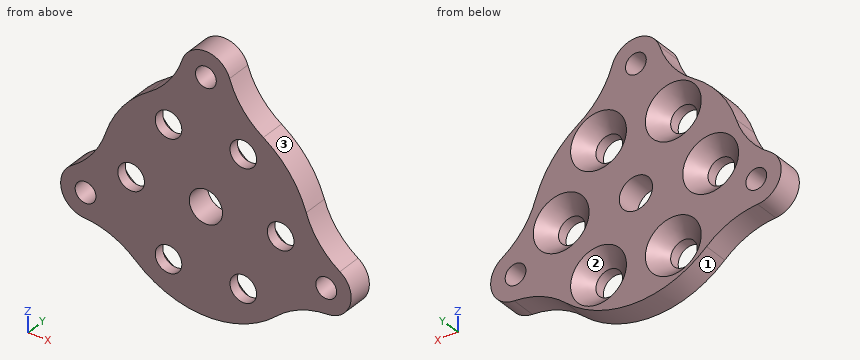
```python
from build123d import *

# Parameters (mm, degrees)
SKETCH1_R                    = 12.7
SKETCH1_R_2                  = 2
BOSS_EXTRUDE1_DEPTH          = 3
CSK_FOR_M3_SFHCS1_AT_2_COUNT = 2
CSK_FOR_M3_SFHCS1_AT_2_PITCH = 9
CSK_FOR_M3_SFHCS1_AT_3_COUNT = 2
CSK_FOR_M3_SFHCS1_AT_3_PITCH = 15.588457268
CSK_FOR_M3_SFHCS1_AT_4_COUNT = 2
CSK_FOR_M3_SFHCS1_AT_4_PITCH = 18
CSK_FOR_M3_SFHCS1_AT_5_COUNT = 2
CSK_FOR_M3_SFHCS1_AT_5_PITCH = 15.588457268
CSK_FOR_M3_SFHCS1_AT_6_COUNT = 2
CSK_FOR_M3_SFHCS1_AT_6_PITCH = 9
SKETCH6_R                    = 3
BOSS_EXTRUDE2_DEPTH          = 3
FILLET1_R                    = 10
TAP_DRILL_FOR_M3X0_5_TAP1_D  = 2.5


with BuildPart() as part:
    # Sketch1 → Boss-Extrude1 (new body)
    with BuildSketch(Plane(origin=(0, 0, 0), x_dir=(1, 0, 0), z_dir=(0, 1, 0))):
        with Locations(Location((0, 0, 0), (0, 0, 270))):
            Circle(SKETCH1_R)
        with Locations(Location((0, 0, 0), (0, 0, 270))):
            Circle(SKETCH1_R_2, mode=Mode.SUBTRACT)
    extrude(amount=BOSS_EXTRUDE1_DEPTH)

    # Sketch3 → CSK for M3 SFHCS1 (revolve, cut)
    with BuildSketch(Plane(origin=(-9, 3, 0), x_dir=(0, 0, 1), z_dir=(1, 0, 0))):
        Polygon((0, 0), (0, 3), (1.6, 3), (1.6, 1.76), (3.36, 0), align=None)
    csk_for_m3_sfhcs1 = revolve(axis=Axis((-9, 9.35, 0), (0, -1, 0)), mode=Mode.SUBTRACT)

    # CSK for M3 SFHCS1 at 2: CSK for M3 SFHCS1 ×2
    with Locations(*[Vector(0.5000000000000003, 0, -0.8660254037844386) * (i * CSK_FOR_M3_SFHCS1_AT_2_PITCH) for i in range(1, CSK_FOR_M3_SFHCS1_AT_2_COUNT)]):
        add(csk_for_m3_sfhcs1, mode=Mode.SUBTRACT)

    # CSK for M3 SFHCS1 at 3: CSK for M3 SFHCS1 ×2
    with Locations(*[Vector(0.8660254037844387, 0, -0.4999999999999999) * (i * CSK_FOR_M3_SFHCS1_AT_3_PITCH) for i in range(1, CSK_FOR_M3_SFHCS1_AT_3_COUNT)]):
        add(csk_for_m3_sfhcs1, mode=Mode.SUBTRACT)

    # CSK for M3 SFHCS1 at 4: CSK for M3 SFHCS1 ×2
    with Locations(*[(i * CSK_FOR_M3_SFHCS1_AT_4_PITCH, 0, 0) for i in range(1, CSK_FOR_M3_SFHCS1_AT_4_COUNT)]):
        add(csk_for_m3_sfhcs1, mode=Mode.SUBTRACT)

    # CSK for M3 SFHCS1 at 5: CSK for M3 SFHCS1 ×2
    with Locations(*[Vector(0.8660254037844387, 0, 0.49999999999999994) * (i * CSK_FOR_M3_SFHCS1_AT_5_PITCH) for i in range(1, CSK_FOR_M3_SFHCS1_AT_5_COUNT)]):
        add(csk_for_m3_sfhcs1, mode=Mode.SUBTRACT)

    # CSK for M3 SFHCS1 at 6: CSK for M3 SFHCS1 ×2
    with Locations(*[Vector(0.5000000000000002, 0, 0.8660254037844386) * (i * CSK_FOR_M3_SFHCS1_AT_6_PITCH) for i in range(1, CSK_FOR_M3_SFHCS1_AT_6_COUNT)]):
        add(csk_for_m3_sfhcs1, mode=Mode.SUBTRACT)

    # Sketch6 → Boss-Extrude2 (add)
    with BuildSketch(Plane(origin=(0, 3, 0), x_dir=(1, 0, 0), z_dir=(0, 1, 0))):
        with Locations((14.488887394, 3.882285677)):
            Circle(SKETCH6_R)
        with Locations((0, -15)):
            Circle(SKETCH6_R)
        with Locations((-14.488887394, 3.882285677)):
            Circle(SKETCH6_R)
    extrude(amount=-BOSS_EXTRUDE2_DEPTH)

    # Fillet1
    fillet1_edges = [part.edges().sort_by_distance(p)[0] for p in [
        (11.690211932, 1.5, -4.962755785),
        (12.605398401, 1.5, -1.547233383),
        (1.768004493, 1.5, 12.576333333),
        (-1.768004493, 1.5, 12.576333333),
        (-11.690211932, 1.5, -4.962755785),
        (-12.605398401, 1.5, -1.547233383),
    ]]
    fillet(fillet1_edges, radius=FILLET1_R)

    # Tap Drill for M3x0.5 Tap1 (through all)
    with Locations(Plane(origin=(0, 3, 0), x_dir=(1, 0, 0), z_dir=(0, 1, 0))):
        with Locations((-14.488887394, 3.882285677), (14.488887394, 3.882285677), (0, -15)):
            Hole(TAP_DRILL_FOR_M3X0_5_TAP1_D / 2)


solid = part.part
```
Design review of the part built by this model. Coordinates are the model's own, in mm. Face numbers are marked on the shaded views. Coordinates: 2 decimals unless noted, no trailing zeros. Order: outer loops, then holes, each group sorted by start corner. A loop starts at its lowest first (then second) coordinate and runs counter-clockwise, first axis right, second up. Notation, with made-up numbers: (67, 30.25) -> (119, 30.25) arc R14 ccw to (119, 35.25) -> close; hole circle Ø10 at (10, 84). An arc over 180 degrees is marked (long way). One line per item, written item: value. Start each with the question number.
Q1. Mouldability with a two-part tool opening along X and no side actions: class the marked faces 1, 2 and 3 as pulls with the +X half, pulls with the -X half, needs draft (parallel to the pull), parting line crosses it, or undercut.
Q2. For probe 1 along Z at (x, y) = (-4, 0.2); probe 2 along X at (y, z) = (2.45, -3.5); probe 3 along X at (y, z) = (1.8, 1.5), list the stretches that pass through material, from the lowest coordinate up.
Q3. Take a section at B-B, the plane z = 0. Give the number of separate pieces and of enclosed holes in the cut face, then the cut area to 3 significant figures.
Q4. Take a section at A-A, the plane x = 0. State the section outline as (y, z) points.
Q5. Insertion check: pin 1 Ø1 at (y, z) = (2.5, 2) entering from -X; pin 2 Ø5 at (x, z) = (4.5, -7.79) entering from +Y; pin 3 Ø4 at (x, z) = (4.5, 7.79) entering from +Y. Each pin has a flat end and moves straight along its axis. Give the tip position at first contact, or say it passes through.
Values follow:
1. face 1: parting line crosses it
1. face 2: undercut
1. face 3: pulls with the +X half
2. probe 1: z = -12.05 to -9.31, -6.27 to 6.27, 9.31 to 13.55
2. probe 2: x = -17.46 to -15.68, -13.3 to 13.3, 15.68 to 17.46
2. probe 3: x = -13.24 to -10.55, -7.45 to -1.32, 1.32 to 7.45, 10.55 to 13.24
3. separate pieces: 4
3. enclosed holes: 0
3. area: 49.3 mm2
4. outline: (0, -12.7) -> (3, -12.7) -> (3, -2) -> (0, -2) -> close; (0, 2) -> (3, 2) -> (3, 13.75) -> (0, 13.75) -> close; (0, 16.25) -> (3, 16.25) -> (3, 18) -> (0, 18) -> close
5. pin 1: stops at x = -13.24
5. pin 2: stops at y = 2.14
5. pin 3: stops at y = 1.64
